Verification items for the finished model (mm, model axes). Give positions to 0.01 mm unless a question says otherwise; leave off trailing zeros. Write each loop counter-clockwise with the first axis right and the second up, starting at its lowest first coordinate (ties: lowest second). Pieces come first, ordered by that corner, then holes. Notation, with made-up numbers: M 42,84 L 68,84 A33 cw 68,117 Z; hole C 41.5,76.5 d11. An arc over 180 degrees is marked long. Answer as a JSON object with one key per item and string values.
```python
from build123d import *

# Parameters (mm, degrees)
F0_W     = 185.286317
F0_H     = 69.482369
F1_DEPTH = 25.4
F2_R     = 10.16


with BuildPart() as f1:
    # F0 (on Top) → F1 (new body, symmetric)
    with BuildSketch(Plane.XY):
        with Locations((32.635657, -10.176711)):
            Rectangle(F0_W, F0_H)
    extrude(amount=F1_DEPTH, both=True)

    # F2
    f2_edges = [f1.edges().sort_by_distance(p)[0] for p in [
        (32.635657, -44.917896, 25.4),
        (32.635657, 24.564473, 25.4),
        (32.635657, -44.917896, -25.4),
        (32.635657, 24.564473, -25.4),
    ]]
    fillet(f2_edges, radius=F2_R)


solid = f1.part
```
1) Section check A-A on x = 19. Record the boundary of the cut face in (y, z).
Completed:
{"outline": "M -44.92,-15.24 A10.16 ccw -34.76,-25.4 L 14.4,-25.4 A10.16 ccw 24.56,-15.24 L 24.56,15.24 A10.16 ccw 14.4,25.4 L -34.76,25.4 A10.16 ccw -44.92,15.24 Z"}
2) Section check C-C on y = -40. Record the boundary of the cut face in (x, z).
Completed:
{"outline": "M -60.01,-23.94 L 125.28,-23.94 L 125.28,23.94 L -60.01,23.94 Z"}
3) Thickness scan on L1, parallel to Y at x = -53, z = -15.5; L2, parallel to Z at x = -4, y = -36.5; L3, parallel to Z at x = 18, y = -40. Record the ranges inside material, lowest first.
Completed:
{"L1": "y = -44.91 to 24.56", "L2": "z = -25.25 to 25.25", "L3": "z = -23.94 to 23.94"}
4) Section check B-B on z = -19.5. Record the boundary of the cut face in (x, y), and give its area (3 significant figures).
Completed:
{"outline": "M -60.01,-43.98 L 125.28,-43.98 L 125.28,23.63 L -60.01,23.63 Z", "area": "12,500 mm2"}
